from build123d import *

# Parameters (mm, degrees)
F0_W        = 88.9
F0_H        = 10.8020305634
F1_DEPTH    = 25.4
F3_W        = 88.9
F3_H        = 10.8020305634
F3_H_2      = 78.0979694366
F4_DEPTH    = 3.81
F5_W        = 88.9
F5_H        = 5.08
F6_DEPTH    = 3.048
F7_T1_DEPTH = 113.4934442484
F7_T3_DEPTH = 114.3
F8_R        = 1.27
F9_R        = 2.032


# Not quite as in the source:
# - a fillet or chamfer that OpenCascade refuses, or shapes differently, is made with other operations: its cross-section is extruded or revolved along the edge and cut away or added
# - a feature names something its author has since deleted; it is built from what else it names


with BuildPart() as f1:
    # F0 (on Front) → F1 (new body)
    with BuildSketch(Plane.XZ):
        with Locations((7.6519327545, -42.832814157)):
            Rectangle(F0_W, F0_H)
    extrude(amount=F1_DEPTH)

    # F3 (on face) → F4 (join)
    with BuildSketch(Plane(origin=(0, 0, 0), x_dir=(-1, 0, 0), z_dir=(0, 1, 0))):
        with Locations((-7.6519327545, -42.832814157)):
            Rectangle(F3_W, F3_H)
        with Locations((-7.6519327545, 1.617185843)):
            Rectangle(F3_W, F3_H_2)
    extrude(amount=F4_DEPTH)

    # F5 (on face) → F6 (cut)
    with BuildSketch(Plane.XY.offset(-37.4317988753)):
        with Locations((7.6519327545, -14.0730550206)):
            Rectangle(F5_W, F5_H)
    extrude(amount=-F6_DEPTH, mode=Mode.SUBTRACT)

    # F7: fillet of radius 5.08 on 4 edges, made by hand

    # F7_s2 → F7_t1 (cut)
    with BuildSketch(Plane.YZ.offset(-49.0947893697)):
        with BuildLine():
            ThreePointArc((0, 35.7474817116), (1.0639073716, 38.858333685), (3.81, 40.6661705613))
            Line((3.81, 40.6661705613), (0, 40.6661705613))
            Line((0, 40.6661705613), (0, 35.7474817116))
        make_face()
    extrude(amount=F7_T1_DEPTH, mode=Mode.SUBTRACT)

    # F7_s4 → F7_t3 (cut)
    with BuildSketch(Plane.YZ.offset(-49.4980672455)):
        with BuildLine():
            ThreePointArc((-25.4, -42.5117988753), (-23.9121024484, -38.9196964269), (-20.32, -37.4317988753))
            Line((-20.32, -37.4317988753), (-25.4, -37.4317988753))
            Line((-25.4, -37.4317988753), (-25.4, -42.5117988753))
        make_face()
        with BuildLine():
            ThreePointArc((-20.32, -48.2338294387), (-23.9121024484, -46.7459318871), (-25.4, -43.1538294387))
            Line((-25.4, -43.1538294387), (-25.4, -48.2338294387))
            Line((-25.4, -48.2338294387), (-20.32, -48.2338294387))
        make_face()
        with BuildLine():
            ThreePointArc((3.81, -43.1538294387), (2.3221024484, -46.7459318871), (-1.27, -48.2338294387))
            Line((-1.27, -48.2338294387), (3.81, -48.2338294387))
            Line((3.81, -48.2338294387), (3.81, -43.1538294387))
        make_face()
    extrude(amount=F7_T3_DEPTH, mode=Mode.SUBTRACT)

    # F8
    f8_edges = [f1.edges().sort_by_distance(p)[0] for p in [
        (7.651933, 3.81, 40.666171),
    ]]
    fillet(f8_edges, radius=F8_R)

    # F9
    f9_edges = [f1.edges().sort_by_distance(p)[0] for p in [
        (7.651933, -16.613055, -40.479799),
        (7.651933, -11.533055, -40.479799),
    ]]
    fillet(f9_edges, radius=F9_R)


solid = f1.part
Read the model definition and answer for the solid it produces. Units are mm, in the model's axes. A direction names the side the tool comes from. Coordinates: 2 decimals unless noted, no trailing zeros. Loops run counter-clockwise (first coordinate to the right, second up) from the corner with the lowest first, then second, coordinate; pieces in that order, holes last.
Q1. The part is cut by section B-B on y = -3.25. Write down the section's boundary in (x, z).
Q2. The part is cut by section C-C on z = -15. Write down the section's boundary in (x, y), and give its area (3 significant figures).
Q3. Consider probe 1 along Z at (x, y) = (2, -11.5); probe 2 along Y at (x, z) = (-1.5, -9); probe 3 along Y at (x, z) = (-6, -38). Determine where each line is inside the solid, lowest interval first.
Q4. The part is cut by section A-A on x = -6. Write down the section's boundary in (y, z), and give its area (3 significant figures).
Q5. Each of these flat-tipped pins is pushed along its axis until it touches: pin 1 Ø8 at (x, y) = (17, -18.5) entering from +Z; pin 2 Ø1.1 at (x, z) = (-3.5, -38) entering from -Y; pin 3 Ø0.8 at (x, y) = (1, -14) entering from +Z. Where does it stop, or does it pass through?
Q6. Which of the six approach directions +Z, -Z, +X, -X, +Y, -Y give full straight-line access (tool end or side, diameter ignored) to faces 1 (the face through (7, -6, -37.432)), 2 (the face through (8.274, -12.113, -39.869)), 3 (the face through (7.03, -23.87, -46.79))?
Q7. The mould has two halves that part along Y. Classify faces 4 (the face through (52.102, 1, -24)), 5 (the face through (8.3, -16, -39.9)), 6 (the face through (8, 3.81, -2)): +Y half, -Y half, draft (parallel to the pull), parting line (faces both ways), or undercut.
Results below:
1. outline: (-36.8, -48.23) - (52.1, -48.23) - (52.1, -37.43) - (-36.8, -37.43) - close
2. outline: (-36.8, 0) - (52.1, 0) - (52.1, 3.81) - (-36.8, 3.81) - close
2. area: 339 mm2
3. probe 1: z = -48.23 to -37.43
3. probe 2: y = 0 to 3.81
3. probe 3: y = -22.65 to -16.61, -11.53 to 3.81
4. outline: (-25.4, -43.15) arc R5.08 ccw to (-20.32, -48.23) - (-1.27, -48.23) arc R5.08 ccw to (3.81, -43.15) - (3.81, 38.59) arc R1.27 ccw to (1.69, 39.53) arc R5.08 ccw to (0, 35.75) - (0, -37.43) - (-11.53, -37.43) - (-11.53, -38.45) arc R2.03 cw to (-13.57, -40.48) - (-14.58, -40.48) arc R2.03 cw to (-16.61, -38.45) - (-16.61, -37.43) - (-20.32, -37.43) arc R5.08 ccw to (-25.4, -42.51) - close
4. area: 577 mm2
5. pin 1: stops at z = -37.43
5. pin 2: stops at y = -23.5
5. pin 3: stops at z = -40.48
6. face 1: +Z, +X, -X, -Y
6. face 2: +Z, +X, -X
6. face 3: -Z, +X, -X, -Y
7. face 4: draft
7. face 5: undercut
7. face 6: +Y half
